Could you check a few things on this model? Use its own coordinates, in mm. Round coordinates to 2 decimals unless told otherwise and drop trailing zeros. Loops run counter-clockwise (first coordinate to the right, second up) from the corner with the lowest first, then second, coordinate; pieces in that order, holes last.
Autodesk Inventor part; units mm, degrees
ref_plane "YZ Plane" through (0, 0, 0) normal (1, 0, 0) x (0, 1, 0)
ref_plane "XZ Plane" through (0, 0, 0) normal (0, 1, 0) x (-1, 0, 0)
ref_plane "XY Plane" through (0, 0, 0) normal (0, 0, 1) x (1, 0, 0)
sketch "Sketch1" plane through (0, 0, 0) normal (0, 1, 0) x (-1, 0, 0)
  line L0 (0, 0) -> (0, -322.934) construction
  line L1 (5, 0) -> (5, -322.934)
  line L2 (-5, -322.934) -> (-5, 0)
  arc A0 (5, 0) -> (-5, 0) centre (0, 0) ccw
  arc A1 (-5, -322.934) -> (5, -322.934) centre (0, -322.934) ccw
  circle A2 centre (0, 0) radius 1.65
  circle A3 centre (0, -322.934) radius 1.65
  circle A4 centre (0, -74.182) radius 1.65
  circle A5 centre (0, -218.733) radius 1.65
  arc A6 (5, -74.182) -> (5, -218.733) centre (600.631, -146.4575) ccw
  arc A7 (-5, -74.182) -> (-5, -218.733) centre (590.631, -146.4575) ccw
  point P0 (0, -161.467)
  dimension "d0" = 3.3
  dimension "d1" = 3.3
  dimension "d2" = 10
  dimension "d3" = 322.934
  dimension "d4" = 3.3
  dimension "d5" = 74.182
  dimension "d8" = 3.3
  dimension "d9" = 218.733
  dimension "d12" = 600
  dimension "d13" = 600
extrude "Extrusion1" add sketch "Sketch1" along normal blind 3 contours L1 A6 A1 L2 A0 | L2 A7
sketch "Sketch2" plane through (0, 3, 0) normal (0, 1, 0) x (1, 0, 0)
  line L0 (-80.742, 377.6004) -> (86.5972, 377.6004)
  line L1 (86.5972, 377.6004) -> (86.5972, -99.7148)
  line L2 (86.5972, -99.7148) -> (-80.742, -99.7148)
  line L3 (-80.742, -99.7148) -> (-80.742, 377.6004)
  line L4 (-25.6776, 342.7032) -> (34.5594, 342.7032)
  line L5 (34.5594, 342.7032) -> (34.5594, 151.6448)
  line L6 (34.5594, 151.6448) -> (-25.6776, 151.6448)
  line L7 (-25.6776, 151.6448) -> (-25.6776, 342.7032)
  point P0 (0, 0)
extrude "Extrusion2" cut sketch "Sketch2" against normal blind 100 contours L4 L5 L6 L7
properties part number "Part_3_p1"
Item 1: If we section it at A-A, the plane y = 0.95: Please give me the cut outline in (x, z).
Results list:
outline: (-5, -74.18) arc R600 cw to (-0.65, -151.64) - (9.35, -151.64) arc R600 ccw to (5, -74.18) - (5, 0) arc R5 ccw to (-5, 0) - close; hole circle Ø3.3 at (0, -74.18); hole circle Ø3.3 at (0, 0)
Item 2: If we section it at B-B, the plane z = -56.5: Please give me the cut outline in (x, y).
Results list:
outline: (-5, 0) - (5, 0) - (5, 3) - (-5, 3) - close
Item 3: Will this pin go through, and if not, where does the flat tip stop? pin 1 (1.5 mm diameter, centred on x = -1.5, y = 2.5, fed in from +Z).
Results list:
pin 1: stops at z = 4.94
Item 4: We'd pull the mould along Z, two halves only. Please class faces 1 (the cylindrical face through (0, 1, 5)), 2 (the cylindrical face through (1.216, 1.479, -1.115)), 3 (the flat face through (5, 1, -38)), 4 (the cylindrical face through (0.21, 1.48, -75.82)): released by +Z, released by -Z, zero draft, split by the parting line, or undercut.
Results list:
face 1: released by +Z
face 2: undercut
face 3: zero draft
face 4: undercut
Item 5: If I drill on line 1 along Z through (x, y) = (0, 1.4); line 2 along X through (y, z) = (2.45, -57); line 3 along X through (y, z) = (1, -142.5), over which ranges is the centre line in solid material (lowest first)?
Results list:
line 1: z = -151.64 to -75.83, -72.53 to -1.65, 1.65 to 5
line 2: x = -5 to 5
line 3: x = -0.64 to 9.36
